from build123d import *

# Parameters (mm, degrees)
SKETCH_1_R               = 7.179803271
EXTRUDE_1_DEPTH          = 50
SKETCH_3_OUTSIDE_W       = 79.114
SKETCH_3_OUTSIDE_H       = 69.114
SKETCH_3_OUTSIDE_R       = 2.5
CUT_EXTRUDE_1_DEPTH      = 17.970562748
CUT_EXTRUDE_1_DEPTH_BACK = 19


with BuildPart() as part:
    # Эскиз1 → Бобышка-Вытянуть1 (new body)
    with BuildSketch(Plane(origin=(0, 0, 0), x_dir=(1, 0, 0), z_dir=(0, 1, 0))):
        with BuildLine():
            Line((-30, 12.727922061), (-30, 6))
            Line((-30, 6), (-16.963843494, 6))
            ThreePointArc((-16.963843494, 6), (-17.993665165, 0), (-16.963843494, -6))
            Line((-16.963843494, -6), (-30, -6))
            Line((-30, -6), (-30, -12))
            Line((-30, -12), (-12, -12))
            ThreePointArc((-12, -12), (0, -16.970562748), (12, -12))
            Line((12, -12), (30, -12))
            Line((30, -12), (30, -6))
            Line((30, -6), (16.963843494, -6))
            ThreePointArc((16.963843494, -6), (17.993665165, 0), (16.963843494, 6))
            Line((16.963843494, 6), (30, 6))
            Line((30, 6), (30, 12.727922061))
            Line((30, 12.727922061), (12.727922061, 12.727922061))
            ThreePointArc((12.727922061, 12.727922061), (0, 18), (-12.727922061, 12.727922061))
            Line((-12.727922061, 12.727922061), (-30, 12.727922061))
        make_face()
        Circle(SKETCH_1_R, mode=Mode.SUBTRACT)
    extrude(amount=EXTRUDE_1_DEPTH)

    # Эскиз3 outside → Вырез-Вытянуть1 (cut, two sides)
    with BuildSketch(Plane.XY) as cut_extrude_1_sk:
        with Locations((0, 25)):
            Rectangle(SKETCH_3_OUTSIDE_W, SKETCH_3_OUTSIDE_H)
        Polygon((21, 50), (-21, 50), (-30, 42.791951294), (-30, 37.841695699), (-21, 30.220907479), (-12, 30.220907479), (-12, 0), (12, 0), (12, 30.220907479), (21, 30.220907479), (30, 37.841695699), (30, 42.791951294), align=None, mode=Mode.SUBTRACT)
        with Locations((-21, 40.381958439)):
            Circle(SKETCH_3_OUTSIDE_R)
        with Locations((21, 40.381958439)):
            Circle(SKETCH_3_OUTSIDE_R)
    extrude(amount=CUT_EXTRUDE_1_DEPTH, mode=Mode.SUBTRACT)
    extrude(cut_extrude_1_sk.sketch, amount=-CUT_EXTRUDE_1_DEPTH_BACK, mode=Mode.SUBTRACT)


solid = part.part
Source: CAD feature listing. Evaluate the final solid. Frame: model axes, mm. A direction names the side the tool comes from. Coordinates: 2 decimals unless noted, no trailing zeros. Loops run counter-clockwise (first coordinate to the right, second up) from the corner with the lowest first, then second, coordinate; pieces in that order, holes last. Notation, with made-up numbers: M 48.25,57.5 L 55.25,57.5 A19 ccw 55.25,67.5 Z; hole C 82,59.5 d2. An arc over 180 degrees is marked long. Answer in a Markdown table with one row per item.
Q1. Section B-B on x = 0. Return the cut outline in (y, z).
Answers below:
| item | result |
|---|---|
| outline | M 0,-18 L 50,-18 L 50,-7.18 L 0,-7.18 Z; M 0,7.18 L 50,7.18 L 50,16.97 L 0,16.97 Z |
Q2. Section C-C on y = 11.5. Return the cut outline in (x, z), plus the area to 3 significant figures.
Answers below:
| item | result |
|---|---|
| outline | M -12,-13.42 A18 ccw 12,-13.42 L 12,12 A16.97 ccw -12,12 Z; hole C 0,0 d14.36 |
| area | 606 mm^2 |
Q3. Set-up query: faces 5 (the flat face through (12, 15, -1)), 6 (the flat face through (30, 40, -9)), 7 (the flat face through (-19, 38, 12)). Return all of +Z, -Z, +X, -X, +Y, -Y with unobstructed straight access to the full face (end or side cutting, diameter ignored); none if empty.
Answers below:
| item | result |
|---|---|
| face 5 | +Z, -Z, +X, -Y |
| face 6 | +Z, -Z, +X, +Y, -Y |
| face 7 | +Z, -X, +Y, -Y |
Q4. Ray query, probe 1 along Y at (x, z) = (21, 10); probe 2 along Z at (x, y) = (27.5, 41); probe 3 along X at (y, z) = (23, 0.5). Return the intervals inside material, ascending. Write a range as from..to.
Answers below:
| item | result |
|---|---|
| probe 1 | y = 30.22..37.88, 42.88..50 |
| probe 2 | z = -12.73..-6, 6..12 |
| probe 3 | x = -12..-7.16, 7.16..12 |
Q5. First-contact query: pin 1 (6.5 mm diameter, centred on x = 23.5, y = 44.5, fed in from -Z); pin 2 (20 mm diameter, centred on x = -24, y = 36.5, fed in from +Z); pin 3 (8 mm diameter, centred on x = 12.5, y = 30.5, fed in from +Z). Flat tips, straight axial feed; report the tip coordinate or a pass-through.
Answers below:
| item | result |
|---|---|
| pin 1 | stops at z = -12.73 |
| pin 2 | stops at z = 12 |
| pin 3 | stops at z = 14.69 |
Q6. Draft query along Z for faces 1 (the flat face through (18.9, 42.2, 12)), 2 (the flat face through (-24, 40, -6)), 3 (the cylindrical face through (-21.54, 37.94, 8.96)), 4 (the cylindrical face through (17.993, 39.972, 0.086)). Return one class per face: pulls with the +Z half, pulls with the -Z half, needs draft (parallel to the pull), parting line crosses it, or undercut.
Answers below:
| item | result |
|---|---|
| face 1 | pulls with the +Z half |
| face 2 | undercut |
| face 3 | needs draft |
| face 4 | undercut |
Q7. Section A-A on z = 0. Return the cut outline in (x, y).
Answers below:
| item | result |
|---|---|
| outline | M -17.99,30.22 L -12,30.22 L -12,0 L -7.18,0 L -7.18,50 L -17.99,50 Z; M 7.18,0 L 12,0 L 12,30.22 L 17.99,30.22 L 17.99,50 L 7.18,50 Z |
Q8. Section D-D on x = -14. Return the cut outline in (y, z).
Answers below:
| item | result |
|---|---|
| outline | M 30.22,-12.73 L 50,-12.73 L 50,12 L 30.22,12 Z |
